from build123d import *

# Parameters (mm, degrees)
F1_R     = 6
F4_R     = 5.05
F5_DEPTH = 20
F6_R     = 5.05
F7_DEPTH = 20


with BuildPart() as f3:
    # F3: sweep along a path in F0
    with BuildLine(Plane.XY) as f3_path:
        Line((-8.6471897678, 0), (-8.6471897678, 20))
        ThreePointArc((-8.6471897678, 20), (-11.5761219559, 27.0710678119), (-18.6471897678, 30))
        Line((-18.6471897678, 30), (-38.6471897678, 30))
    # F1 (on Front) → F3 (sweep)
    with BuildSketch(Plane.XZ):
        with Locations((-8.6471897678, 0)):
            Circle(F1_R)
    sweep(path=f3_path.line)

    # F4 (on face) → F5 (cut)
    with BuildSketch(Plane.XZ):
        with Locations((-8.6471897678, 0)):
            Circle(F4_R)
    extrude(amount=-F5_DEPTH, mode=Mode.SUBTRACT)

    # F6 (on face) → F7 (cut)
    with BuildSketch(Plane(origin=(-38.6471897678, 0, 0), x_dir=(0, -1, 0), z_dir=(-1, 0, 0))):
        with Locations((-30, 0)):
            Circle(F6_R)
    extrude(amount=-F7_DEPTH, mode=Mode.SUBTRACT)


solid = f3.part
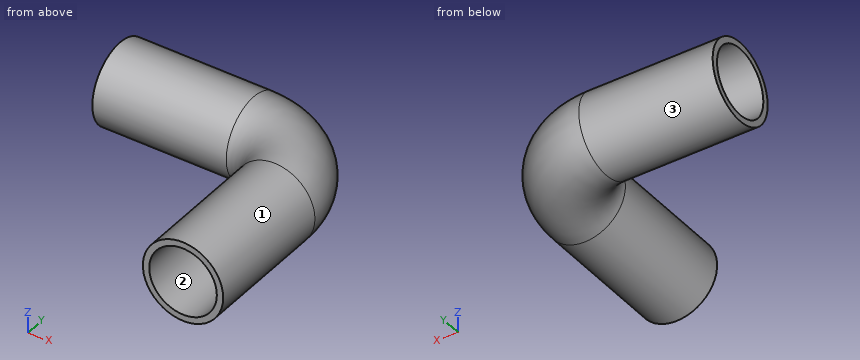
Can you work these out from the model? Positions are in its coordinate system, mm. Face numbers are marked on the shaded views. Coordinates: 2 decimals unless noted, no trailing zeros. Order: outer loops, then holes, each group sorted by start corner. A loop starts at its lowest first (then second) coordinate and runs counter-clockwise, first axis right, second up. Notation, with made-up numbers: (43.25, 33) -> (62.25, 33) arc R25 ccw to (62.25, 54) -> close; hole circle Ø2 at (-40, -3.75). An arc over 180 degrees is marked (long way). Use one line per item in the form item = value.
Q1. We'd pull the mould along X, two halves only. Please class the marked faces 1, 2 and 3: released by +X, released by -X, zero draft, split by the parting line, or undercut.
From the geometry:
face_1 = split by the parting line
face_2 = undercut
face_3 = zero draft
Q2. Imagine slicing it at C-C, the plane x = -33.5. List the corners of the cut face in (y, z) for me, then the cut area to 3 significant figures.
From the geometry:
outline = circle Ø12 at (30, 0); hole circle Ø10.1 at (30, 0)
area = 33.0 mm²
Q3. Imagine slicing it at D-D, the plane z = 0. List the corners of the cut face in (x, y) for me.
From the geometry:
outline = (-38.65, 24) -> (-18.65, 24) arc R4 cw to (-14.65, 20) -> (-14.65, 0) -> (-13.7, 0) -> (-13.7, 20) -> (-3.6, 20) -> (-3.6, 0) -> (-2.65, 0) -> (-2.65, 20) arc R16 ccw to (-18.65, 36) -> (-38.65, 36) -> (-38.65, 35.05) -> (-18.65, 35.05) -> (-18.65, 24.95) -> (-38.65, 24.95) -> close
Q4. Imagine slicing it at A-A, the plane y = 3. List the corners of the cut face in (x, z) for me, then the cut area to 3 significant figures.
From the geometry:
outline = circle Ø12 at (-8.65, 0); hole circle Ø10.1 at (-8.65, 0)
area = 33.0 mm²
Q5. I need wall thicknesses on L1, parallel to Z at x = -33.25, y = 30; L2, parallel to Z at x = -10.5, y = 14; L3, parallel to X at y = 6, z = -1.5. Which ranges of each line are inside material? Lowest first, please.
From the geometry:
L1 = -6 to -5.05, 5.05 to 6
L2 = -5.71 to -4.7, 4.7 to 5.71
L3 = -14.46 to -13.47, -3.83 to -2.84
Q6. Imagine slicing it at B-B, the plane z = -2.5. List the corners of the cut face in (x, y) for me.
From the geometry:
outline = (-38.65, 24.55) -> (-18.65, 24.55) arc R4.55 cw to (-14.1, 20) -> (-14.1, 0) -> (-13.03, 0) -> (-13.03, 20) -> (-4.26, 20) -> (-4.26, 0) -> (-3.19, 0) -> (-3.19, 20) arc R15.45 ccw to (-18.65, 35.45) -> (-38.65, 35.45) -> (-38.65, 34.39) -> (-18.65, 34.39) -> (-18.65, 25.61) -> (-38.65, 25.61) -> close
Q7. Will these pins go through, and if not, where does the flat tip stop? P1, Ø6, axis at x = -21, z = -4, coming from the -Y side; P2, Ø2, axis at x = -10.5, y = 6.5, coming from the +Z side; P3, Ø3, axis at y = 19, z = -4, coming from the +X side.
From the geometry:
P1 = 24.08
P2 = 5.94
P3 = -3.19
